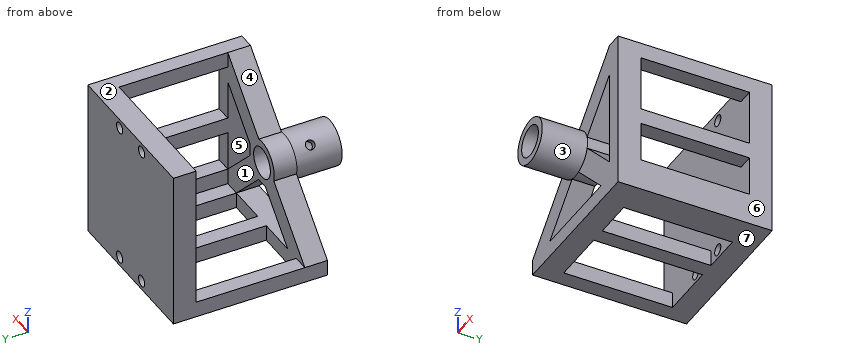
Autodesk Inventor part; units mm, degrees
ref_plane "YZ Plane" through (0, 0, 0) normal (1, 0, 0) x (0, 1, 0)
ref_plane "XZ Plane" through (0, 0, 0) normal (0, 1, 0) x (-1, 0, 0)
ref_plane "XY Plane" through (0, 0, 0) normal (0, 0, 1) x (1, 0, 0)
sketch "Sketch1" plane through (0, 0, 0) normal (0, 1, 0) x (-1, 0, 0)
  line L0 (-17.5, -17.5) -> (17.5, -17.5)
  line L1 (17.5, -17.5) -> (17.5, 17.5)
  line L2 (17.5, 17.5) -> (-17.5, 17.5)
  line L3 (-17.5, 17.5) -> (-17.5, -17.5)
  line L4 (-17.5, -17.5) -> (17.5, 17.5) construction
  line L5 (17.5, -17.5) -> (-17.5, 17.5) construction
  point P0 (0, 0)
  dimension "d0" = 35
  dimension "d1" = 35
extrude "Extrusion1" add sketch "Sketch1" along normal blind 5
sketch "Sketch2" plane through (0, 0, 0) normal (0, -1, 0) x (1, 0, 0)
  circle A0 centre (4.5, 15.5) radius 1.25
  circle A1 centre (-4.5, 15.5) radius 1.25
  circle A2 centre (4.5, -15.5) radius 1.25
  circle A3 centre (-4.5, -15.5) radius 1.25
  point P0 (0, 0)
extrude "Extrusion2" cut sketch "Sketch2" against normal blind 5
sketch "Sketch3" plane through (0, 0, 0) normal (0, -1, 0) x (1, 0, 0)
  line L0 (-17.5, -17.5) -> (-17.5, 17.5)
  line L1 (-17.5, -17.5) -> (-14, -17.5)
  line L2 (-14, -17.5) -> (-14, -14)
  line L3 (-14, -14) -> (-17.5, -14)
  line L4 (-17.5, -14) -> (-17.5, -17.5)
  line L5 (17.5, 17.5) -> (17.5, -17.5)
  line L6 (17.5, -17.5) -> (10.5, -17.5)
  line L7 (10.5, -17.5) -> (10.5, -14)
  line L8 (10.5, -14) -> (17.5, -14)
  line L9 (17.5, -14) -> (17.5, -17.5)
  line L10 (17.5, -14) -> (14, -14)
  line L11 (14, -14) -> (14, -10.5)
  line L12 (14, -10.5) -> (17.5, -10.5)
  line L13 (17.5, -10.5) -> (17.5, -14)
  line L14 (17.5, 17.5) -> (14, 17.5)
  line L15 (14, 17.5) -> (14, 14)
  line L16 (14, 14) -> (17.5, 14)
  line L17 (17.5, 14) -> (17.5, 17.5)
  line L18 (17.5, -17.5) -> (-17.5, -17.5)
  line L19 (1.75, -17.5) -> (-1.75, -17.5)
  line L20 (-1.75, -17.5) -> (-1.75, -14)
  line L21 (-1.75, -14) -> (1.75, -14)
  line L22 (1.75, -14) -> (1.75, -17.5)
  line L23 (17.5, 17.5) -> (17.5, -17.5)
  line L24 (17.5, 1.75) -> (14, 1.75)
  line L25 (14, 1.75) -> (14, -1.75)
  line L26 (14, -1.75) -> (17.5, -1.75)
  line L27 (17.5, -1.75) -> (17.5, 1.75)
  point P0 (0, 0)
  dimension "d6" = 3.5
  dimension "d7" = 3.5
  dimension "d8" = 7
  dimension "d9" = 3.5
  dimension "d10" = 3.5
  dimension "d11" = 3.5
  dimension "d12" = 3.5
  dimension "d13" = 3.5
  dimension "d14" = 3.5
  dimension "d15" = 3.5
  dimension "d16" = 3.5
  dimension "d17" = 3.5
  dimension "d18" = 1.75
  dimension "d19" = 1.75
extrude "Extrusion3" add sketch "Sketch3" along normal blind 24
sketch "Sketch4" plane through (0, -24, 0) normal (0, -1, 0) x (1, 0, 0)
  line L0 (-17.5, -14) -> (-14, -14)
  line L1 (14, 14) -> (14, 17.5)
  line L2 (10.5, -17.5) -> (10.5, -14)
  line L3 (14, -10.5) -> (17.5, -10.5)
  line L4 (-17.5, -14) -> (-17.5, -17.5)
  line L5 (-17.5, -14) -> (-17.5, -17.5)
  line L6 (17.5, 17.5) -> (17.5, -17.5)
  line L7 (-17.5, -17.5) -> (17.5, -17.5)
  line L8 (17.5, -17.5) -> (17.5, 17.5)
  line L9 (17.5, 17.5) -> (14, 17.5)
  line L10 (17.5, 17.5) -> (14, 17.5)
  line L11 (14, -14) -> (10.5, -14)
  line L12 (14, 17.5) -> (14, 14)
  line L13 (-17.5, -14) -> (-4.8221, -1.3221)
  line L14 (1.3221, 4.8221) -> (14, 17.5)
  line L15 (-10.5, -14) -> (-1.3221, -4.8221)
  line L16 (4.8221, 1.3221) -> (14, 10.5)
  line L17 (10.5, -14) -> (7.875, -11.375)
  line L18 (4.375, -7.875) -> (1.3221, -4.8221)
  line L19 (14, -10.5) -> (11.375, -7.875)
  line L20 (7.875, -4.375) -> (4.8221, -1.3221)
  line L21 (-10.5, -14) -> (-1.75, -14)
  line L22 (5.25, -14) -> (10.5, -14)
  circle A0 centre (0, 0) radius 3.415
  arc A1 (-1.3221, -4.8221) -> (1.3221, -4.8221) centre (0, 0) ccw
  arc A2 (4.8221, -1.3221) -> (4.8221, 1.3221) centre (0, 0) ccw
  arc A3 (1.3221, 4.8221) -> (-4.8221, -1.3221) centre (0, 0) ccw
  line L23 (10.5, -14) -> (7.875, -11.375)
  line L24 (10.5, -14) -> (14, -14)
  line L25 (5.25, -14) -> (10.5, -14)
  line L26 (-1.75, -17.5) -> (-1.75, -14)
  line L27 (-1.75, -14) -> (5.25, -14)
  line L28 (14, -1.75) -> (14, 1.75)
  line L29 (7.875, -4.375) -> (11.375, -7.875)
  line L30 (7.875, -11.375) -> (4.375, -7.875)
  line L31 (14, 10.5) -> (14, -10.5)
  point P0 (-14, -17.5)
  point P1 (17.5, 14)
  point P2 (17.5, -1.75)
  dimension "d28" = 6.83
ref_plane "Work Plane1" through (-3.5355, -24, 3.5355) normal (-0.7071068, 0, 0.7071068) x (0, -1, 0)
ref_plane "Work Plane2" through (0, -29, 0) normal (0, -1, 0) x (1, 0, 0)
sketch "Sketch6" plane through (0, -29, 0) normal (0, -1, 0) x (1, 0, 0)
  circle A0 centre (0, 0) radius 3.415
  circle A1 centre (0, 0) radius 5
extrude "Extrusion6" add sketch "Sketch6" along normal blind 10
sketch "Sketch7" plane through (-3.5355, -24, 3.5355) normal (-0.7071068, 0, 0.7071068) x (0, -1, 0)
  circle A0 centre (8.733, 0) radius 1
  point P0 (-24, 0)
  dimension "d31" = 2
extrude "Extrusion7" cut sketch "Sketch7" against normal blind 2
extrude "Extrusion9" add sketch "Sketch4" along normal blind 5 contours L7 L26 L27 L22 L2 | L2 L17 L30 L18 A1 L15 L21 L26 L7 L4 L13 A3 L14 L9 L6
properties part number "Sy_holder"
Design review of the part built by this model. Coordinates are the model's own, in mm. Face numbers are marked on the shaded views. A direction names the side the tool comes from. Give positions to 0.01 mm unless a question says otherwise; leave off trailing zeros. Order: outer loops, then holes, each group sorted by start corner. A loop starts at its lowest first (then second) coordinate and runs counter-clockwise, first axis right, second up.
1. Add section D-D, the plane x = -12. State the section outline as (y, z) points.
Solution:
outline: (-29, -17.5) - (-24, -17.5) - (-24, -8.5) - (-29, -8.5) - close; (0, -17.5) - (5, -17.5) - (5, 17.5) - (0, 17.5) - close
2. To check wall thickness, follow L1, parallel to Z at x = 0, y = -26 (3 decimals); L2, parallel to Z at x = 4.5, y = 1.35; L3, parallel to Y at x = -6.5, z = -6. State the ranges of each line that lie inside material, in increasing order.
Solution:
L1: z = -17.5 to -14, -5 to -3.415, 3.415 to 5
L2: z = -17.5 to -16.75, -14.25 to 14.25, 16.75 to 17.5
L3: y = -29 to -24, 0 to 5
3. Add section B-B, the plane y = -15. State the section outline as (x, z) points.
Solution:
outline: (-17.5, -17.5) - (-14, -17.5) - (-14, -14) - (-17.5, -14) - close; (-1.75, -17.5) - (1.75, -17.5) - (1.75, -14) - (-1.75, -14) - close; (10.5, -17.5) - (17.5, -17.5) - (17.5, -10.5) - (14, -10.5) - (14, -14) - (10.5, -14) - close; (14, -1.75) - (17.5, -1.75) - (17.5, 1.75) - (14, 1.75) - close; (14, 14) - (17.5, 14) - (17.5, 17.5) - (14, 17.5) - close
4. Add section C-C, the plane z = -7. State the section outline as (x, y) points.
Solution:
outline: (-17.5, 0) - (17.5, 0) - (17.5, 5) - (-17.5, 5) - close; (-10.5, -29) - (-3.5, -29) - (-3.5, -24) - (-10.5, -24) - close; (3.5, -29) - (10.5, -29) - (10.5, -24) - (3.5, -24) - close; (14, -29) - (17.5, -29) - (17.5, -24) - (14, -24) - close
5. Mouldability with a two-part tool opening along Z and no side actions: class the marked faces 4, 5, 6 and 7 as +Z half, -Z half, draft (parallel to the pull), parting line (faces both ways), or undercut.
Solution:
face 4: +Z half
face 5: undercut
face 6: draft
face 7: -Z half
6. For pin 1 Ø1 at (x, y) = (-9.5, -27) entering from +Z; pin 2 Ø12 at (y, z) = (-0.5, 7) entering from +X; pin 3 Ø5 at (x, y) = (-3, -27) entering from +Z (3 decimals); pin 4 Ø12 at (y, z) = (-7.5, -3) entering from -X, all flat-tipped, find the tip position at first contact; note any pin that passes through.
Solution:
pin 1: stops at z = -5.5
pin 2: stops at x = 17.5
pin 3: stops at z = 4.975
pin 4: stops at x = 14
7. Add section A-A, the plane x = -8. State the section outline as (y, z) points, then the cut area to 4 significant figures.
Solution:
outline: (-29, -17.5) - (-24, -17.5) - (-24, -14) - (-29, -14) - close; (-29, -11.5) - (-24, -11.5) - (-24, -4.5) - (-29, -4.5) - close; (0, -17.5) - (5, -17.5) - (5, 17.5) - (0, 17.5) - close
area: 227.5 mm2
8. Tool access review of the marked faces 1, 2 and 3: name each direction out of +Z, -Z, +X, -X, +Y, -Y from which nothing blocks a thin tool from reaching the whole face with its end or side.
Solution:
face 1: none
face 2: +Z, +X, -X, +Y, -Y
face 3: -Y
